from build123d import *

# Parameters (mm, degrees)
SKETCH_1_W          = 8
SKETCH_1_H          = 6
EXTRUDE_1_DEPTH     = 17.5
SKETCH_2_R          = 2.5
EXTRUDE_2_DEPTH     = 22.5
FILLET_1_R          = 2
HOLE_WIZARD_M3_1_D  = 2.5
SKETCH_6_R          = 1
CUT_EXTRUDE_1_DEPTH = 24.627314701
HOLE_WIZARD_M3_2_D  = 2.5


with BuildPart() as part:
    # 草圖1 → 填料-伸長1 (new, symmetric)
    with BuildSketch(Plane(origin=(0, 0, 0), x_dir=(0, 0, -1), z_dir=(1, 0, 0))):
        Rectangle(SKETCH_1_W, SKETCH_1_H)
    extrude(amount=EXTRUDE_1_DEPTH, both=True)

    # 草圖2 → 填料-伸長2 (add, symmetric)
    with BuildSketch(Plane(origin=(0, 0, 0), x_dir=(0, 0, -1), z_dir=(1, 0, 0))):
        with Locations(Location((0, 0, 0), (0, 0, 180))):
            Circle(SKETCH_2_R)
    extrude(amount=EXTRUDE_2_DEPTH, both=True)

    # 圓角1
    fillet_1_edges = [part.edges().sort_by_distance(p)[0] for p in [
        (0, 3, 4),
        (0, 3, -4),
        (0, -3, -4),
        (0, -3, 4),
    ]]
    fillet(fillet_1_edges, radius=FILLET_1_R)

    # M3 螺紋孔1 (through all)
    with Locations(Plane(origin=(22.5, 0, 0), x_dir=(0, 0, -1), z_dir=(1, 0, 0))):
        with Locations((0, 0)):
            Hole(HOLE_WIZARD_M3_1_D / 2)

    # 草圖6 → 除料-伸長1 (cut, through all)
    with BuildSketch(Plane(origin=(0, 3, 0), x_dir=(1, 0, 0), z_dir=(0, 1, 0))):
        with Locations(Location((-12.5, 0, 0), (0, 0, 270))):
            Circle(SKETCH_6_R)
        with Locations(Location((12.5, 0, 0), (0, 0, 270))):
            Circle(SKETCH_6_R)
    extrude(amount=-CUT_EXTRUDE_1_DEPTH, mode=Mode.SUBTRACT)

    # M3 螺紋孔2 (through all)
    with Locations(Plane(origin=(-12.5, 3, 0), x_dir=(0, 0, 1), z_dir=(0, 1, 0))):
        with Locations((0, 0), (0, 25)):
            Hole(HOLE_WIZARD_M3_2_D / 2)


solid = part.part
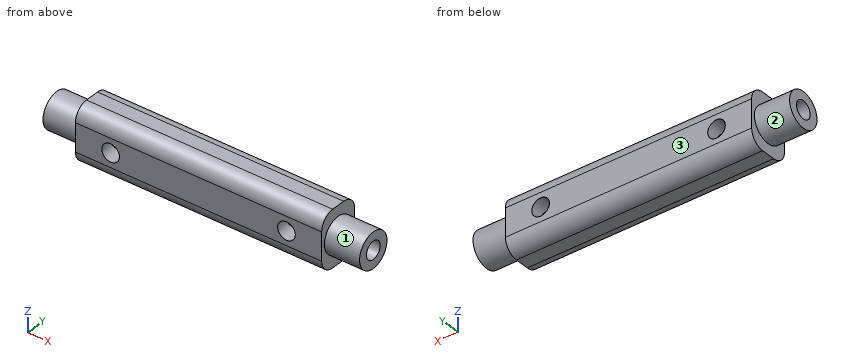
The listing builds one solid part. Answer for the finished solid, in the listing's coordinates (mm). Face numbers are marked on the shaded views. A direction names the side the tool comes from. Round coordinates to 2 decimals unless told otherwise and drop trailing zeros. Write each loop counter-clockwise with the first axis right and the second up, starting at its lowest first coordinate (ties: lowest second). Pieces come first, ordered by that corner, then holes. Notation, with made-up numbers: M 81.25,24 L 88.25,24 A23 ccw 88.25,43 Z; hole C 68,34.25 d1. An arc over 180 degrees is marked long. Write each question's results on one line, items separated by ' | '. Start each with the question number.
Item 1: Straight lines are drawn through the part: L1, parallel to X at y = -2.3, z = 0; L2, parallel to Z at x = -7, y = 0; L3, parallel to X at y = -1.5, z = 0.75. For each, find the intervals that lie inside material, in ascending order. Write a range as [from, to].
Item 2: A cutting plane is placed at C-C on y = -0.5. Write down the section's boundary in (x, z).
Item 3: A flat-ended cylindrical pin translates along its axis: pin 1 Ø2 at (x, z) = (-12.5, 0) entering from -Y. Find the tip coordinate at first contact, or state that the pin passes through.
Item 4: A cutting plane is placed at B-B on x = -1. Write down the section's boundary in (y, z), and give its area (3 significant figures).
Item 5: A cutting plane is placed at A-A on z = 0. State how many separate pieces and enclosed holes the cut face has, and give its area (3 significant figures).
Item 6: A cutting plane is placed at D-D on z = 3. Write down the section's boundary in (x, y).
Item 7: For the marked faces 1, 2 and 3, determine the directions among +Z, -Z, +X, -X, +Y, -Y from which every point of the face is accessible in a straight line to the end or side of a thin tool.
Check sheet entries:
1) L1: [-22.5, -13.75], [-11.25, 11.25], [13.75, 22.5] | L2: [-4, -1.25], [1.25, 4] | L3: [-22.5, -13.5], [-11.5, 11.5], [13.5, 22.5]
2) outline: M -22.5,-2.45 L -17.5,-2.45 L -17.5,-4 L 17.5,-4 L 17.5,-2.45 L 22.5,-2.45 L 22.5,-1.15 L 13,-1.15 A1.25 cw 12,-1.15 L -12,-1.15 A1.25 cw -13,-1.15 L -22.5,-1.15 Z; M -22.5,1.15 L -13,1.15 A1.25 cw -12,1.15 L 12,1.15 A1.25 cw 13,1.15 L 22.5,1.15 L 22.5,2.45 L 17.5,2.45 L 17.5,4 L -17.5,4 L -17.5,2.45 L -22.5,2.45 Z
3) pin 1: through
4) outline: M -3,-2 A2 ccw -1,-4 L 1,-4 A2 ccw 3,-2 L 3,2 A2 ccw 1,4 L -1,4 A2 ccw -3,2 Z; hole C 0,0 d2.5 | area: 39.7 mm²
5) separate pieces: 6 | enclosed holes: 0 | area: 130 mm²
6) outline: M -17.5,-2.73 L 17.5,-2.73 L 17.5,2.73 L -17.5,2.73 Z
7) face 1: +X | face 2: -X | face 3: +Z, -Z, +X, -X, +Y
